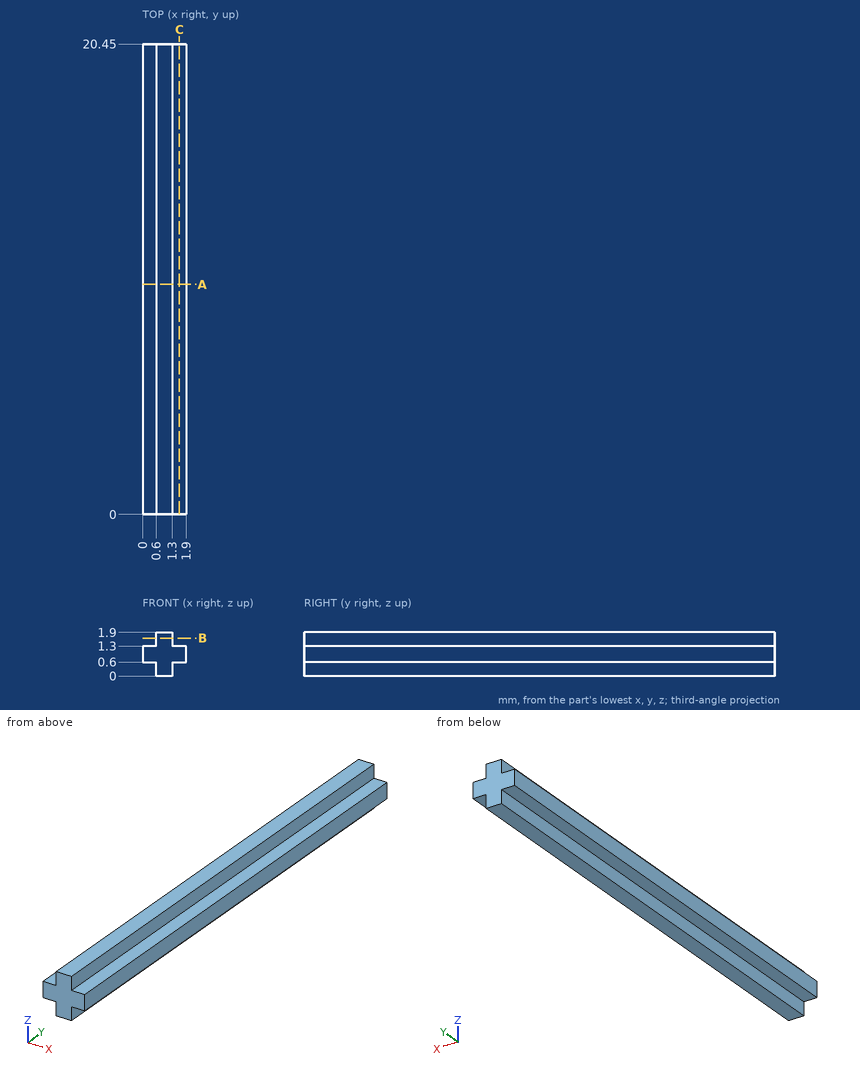
Can you work these out from the drawing? Everything is in mm from the part's minimum corner. Give positions to 0.01 mm unless a question says otherwise; leave off trailing zeros. Loops run counter-clockwise (first coordinate to the right, second up) from the corner with the lowest first, then second, coordinate; pieces in that order, holes last. Notation, with made-up numbers: (27, 87) -> (79, 87) arc R20 ccw to (79, 94) -> close; hole circle Ø10 at (-38, 64.5). An arc over 180 degrees is marked (long way). Return JSON: item names as keys, results as strings.
Item 1: I'm going to push flat-ended pins straight in: pin 1 (1 mm diameter, centred on y = 4, z = 0, fed in from -X); pin 2 (0.7 mm diameter, centred on y = 7, z = 0, fed in from +X); pin 3 (1 mm diameter, centred on y = 8.5, z = 1.5, fed in from +X); pin 4 (0.7 mm diameter, centred on x = 0, y = 5.5, fed in from +Z). Where does each tip first touch, or does it pass through?
Geometry results:
{"pin 1": "stops at x = 0.6", "pin 2": "stops at x = 1.3", "pin 3": "stops at x = 1.9", "pin 4": "stops at z = 1.3"}
Item 2: If we section it at C-C on x = 1.6: List the corners of the cut face in (y, z) for me, plus the area to 3 significant figures.
Geometry results:
{"outline": "(0, 0.6) -> (20.45, 0.6) -> (20.45, 1.3) -> (0, 1.3) -> close", "area": "14.3 mm²"}
Item 3: If we section it at B-B on z = 1.65: List the corners of the cut face in (x, y) for me, plus the area to 3 significant figures.
Geometry results:
{"outline": "(0.6, 0) -> (1.3, 0) -> (1.3, 20.45) -> (0.6, 20.45) -> close", "area": "14.3 mm²"}
Item 4: If we section it at A-A on y = 10: List the corners of the cut face in (x, z) for me, plus the area to 3 significant figures.
Geometry results:
{"outline": "(0, 0.6) -> (0.6, 0.6) -> (0.6, 0) -> (1.3, 0) -> (1.3, 0.6) -> (1.9, 0.6) -> (1.9, 1.3) -> (1.3, 1.3) -> (1.3, 1.9) -> (0.6, 1.9) -> (0.6, 1.3) -> (0, 1.3) -> close", "area": "2.17 mm²"}
Item 5: I need wall thicknesses on L1, parallel to Z at x = 0.3, y = 8.75. Which ranges of the line are inside material? Lowest first, please. Write a range as from..to.
Geometry results:
{"L1": "z = 0.6..1.3"}
